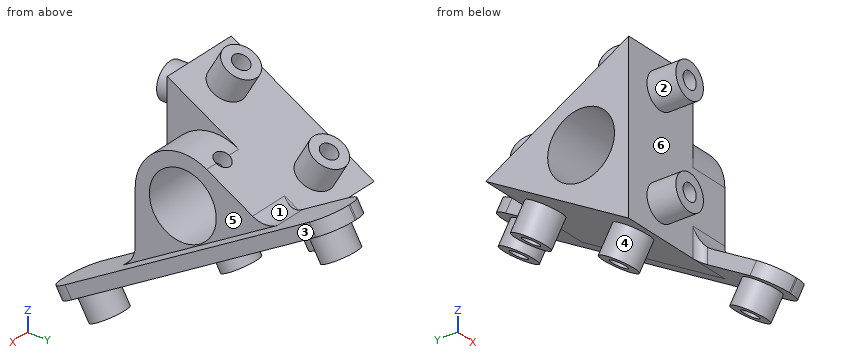
```python
from build123d import *

# Parameters (mm, degrees)
SKETCH_R           = 4.05
PAD_DEPTH          = 15
SKETCH001_R        = 2.15
SKETCH001_R_2      = 1.025
PAD001_DEPTH       = 3.5
POLARPATTERN_COUNT = 3
POLARPATTERN_ANGLE = 240
SKETCH002_R        = 1
POCKET_DEPTH       = 5
SKETCH003_W        = 40
SKETCH003_H        = 6
PAD002_DEPTH       = 1.6
SKETCH004_R        = 2.15
SKETCH004_R_2      = 1.025
PAD003_DEPTH       = 3
POCKET001_DEPTH    = 5
FILLET_R           = 3
FILLET001_R        = 2.9
FILLET002_R        = 1
FILLET003_R        = 1


with BuildPart() as part:
    # Sketch → Pad (new body)
    with BuildSketch(Plane.YZ):
        Polygon((-5.7735026919, 10), (-5.7735026919, -10), (11.5470053838, 0), align=None)
        Circle(SKETCH_R, mode=Mode.SUBTRACT)
    extrude(amount=PAD_DEPTH)

    # Sketch001 (on Face1 of Pad) → Pad001 (join)
    with BuildSketch(Plane(origin=(0, -5.7735026919, 0), x_dir=(0, 0, -1), z_dir=(0, -1, 0))):
        with Locations((6.15, 5)):
            Circle(SKETCH001_R)
        with Locations((6.15, 5)):
            Circle(SKETCH001_R_2, mode=Mode.SUBTRACT)
        with Locations((-6.15, 5)):
            Circle(SKETCH001_R)
        with Locations((-6.15, 5)):
            Circle(SKETCH001_R_2, mode=Mode.SUBTRACT)
    pad001 = extrude(amount=PAD001_DEPTH)

    # PolarPattern: Pad001 ×3 about axis
    polarpattern_axis = Axis((0, 0, 0), (1, 0, 0))
    for i in range(1, POLARPATTERN_COUNT):
        add(pad001.rotate(polarpattern_axis, i * POLARPATTERN_ANGLE / (POLARPATTERN_COUNT - 1)))

    # Sketch002 (on Face2 of PolarPattern) → Pocket (cut)
    with BuildSketch(Plane(origin=(0, 2.8867513459, 5), x_dir=(0, -0.8660254038, 0.5), z_dir=(0, 0.5, 0.8660254038))):
        with Locations((0, 12.5)):
            Circle(SKETCH002_R)
    extrude(amount=-POCKET_DEPTH, mode=Mode.SUBTRACT)

    # Sketch003 (on Face5 of Pocket) → Pad002 (join)
    with BuildSketch(Plane(origin=(0, 2.8867513459, -5), x_dir=(0, 0.8660254038, 0.5), z_dir=(0, 0.5, -0.8660254038))):
        with Locations((0, 14)):
            Rectangle(SKETCH003_W, SKETCH003_H)
    extrude(amount=-PAD002_DEPTH)

    # Sketch004 (on Face14 of Pad002) → Pad003 (join)
    with BuildSketch(Plane(origin=(0, 2.8867513459, -5), x_dir=(0, 0.8660254038, 0.5), z_dir=(0, 0.5, -0.8660254038))):
        with Locations((-16.2, 14)):
            Circle(SKETCH004_R)
        with Locations((-16.2, 14)):
            Circle(SKETCH004_R_2, mode=Mode.SUBTRACT)
        with Locations((16.2, 14)):
            Circle(SKETCH004_R)
        with Locations((16.2, 14)):
            Circle(SKETCH004_R_2, mode=Mode.SUBTRACT)
    extrude(amount=PAD003_DEPTH)

    # Sketch005 (on Face6 of Pad003) → Pocket001 (cut)
    with BuildSketch(Plane.YZ.offset(15)):
        with BuildLine():
            Line((-5.7735026919, 0), (-5.7735026919, 10))
            Line((-5.7735026919, 10), (2.8867345187, 5.0000097152))
            ThreePointArc((2.8867345187, 5.0000097152), (-2.8867597595, 4.9999951424), (-5.7735026919, 0))
        make_face()
    extrude(amount=-POCKET001_DEPTH, mode=Mode.SUBTRACT)

    # Fillet
    fillet_edges = [part.edges().sort_by_distance(p)[0] for p in [
        (13, 9.947005, 0.92376),
        (13, -5.773503, -8.152479),
    ]]
    fillet(fillet_edges, radius=FILLET_R)

    # Fillet001
    fillet001_edges = [part.edges().sort_by_distance(p)[0] for p in [
        (17, -14.833757, -14.30718),
        (11, -14.833757, -14.30718),
        (17, 19.807259, 5.69282),
        (11, 19.807259, 5.69282),
    ]]
    fillet(fillet001_edges, radius=FILLET001_R)

    # Fillet002
    fillet002_edges = [part.edges().sort_by_distance(p)[0] for p in [
        (11, -5.773503, -9.07624),
        (11, -5.773503, -7.286454),
    ]]
    fillet(fillet002_edges, radius=FILLET002_R)

    # Fillet003
    fillet003_edges = [part.edges().sort_by_distance(p)[0] for p in [
        (11, 9.197005, 1.356773),
        (11, 10.747005, 0.46188),
    ]]
    fillet(fillet003_edges, radius=FILLET003_R)


solid = part.part
```
Geometry check sheet. Reference: the model listing, model coordinates, mm. Face numbers are marked on the shaded views. A direction names the side the tool comes from. Give positions to 0.01 mm unless a question says otherwise; leave off trailing zeros. Loops run counter-clockwise (first coordinate to the right, second up) from the corner with the lowest first, then second, coordinate; pieces in that order, holes last. Notation, with made-up numbers: M 18.5,7.5 L 51.5,7.5 A17 cw 51.5,16.5 Z; hole C 65.5,-24.5 d6. An arc over 180 degrees is marked long. Write item = value, one per line. Start each with the question number.
1. Section check C-C, the plane x = 2. Enter the section's corners in (y, z).
2. Go/stop test with flat-tipped pins: P1, Ø1, axis at y = 3.5, z = -7.5, coming from the -X side; P2, Ø3.5, axis at x = 5, z = -5.5, coming from the -Y side; P3, Ø1.2, axis at x = 5, z = -6.15, coming from the -Y side; P4, Ø1.5, axis at x = 4, z = -12.5, coming from the +Y side. Record where each tip stops, or that it passes through.
3. Thickness scan on probe 1 along X at (y, z) = (-8.5, -6.15) (3 decimals); probe 2 along X at (y, z) = (-7, 4.5); probe 3 along X at (y, z) = (-0.5, 4.5). Record the ranges inside material, lowest first.
4. Draft check along Y on the marked faces 4, 5 and 6. Enter one of: +Y half, -Y half, draft (parallel to the pull), parting line (faces both ways), or undercut.
5. Section check A-A, the plane x = 6.5. Enter the section's corners in (y, z), plus the area to 3 significant figures.
6. Section check B-B, the plane y = 13. Enter the section's corners in (x, z), plus the area to 3 significant figures.
7. Tool access check on the marked faces 1, 2 and 3. Record the directions out of +Z, -Z, +X, -X, +Y, -Y that give a thin tool (end or side, any length) a straight path to the whole face; none if there is none.
Values follow:
q1.outline = M -5.77,-10 L 11.55,0 L -5.77,10 Z; hole C 0,0 d8.1
q2.P1 = through
q2.P2 = -9.27
q2.P3 = -5.77
q2.P4 = -1.8
q3.probe_1 = 2.85 to 3.975, 6.025 to 7.15
q3.probe_2 = 3.62 to 6.38
q3.probe_3 = 0 to 15
q4.face_4 = undercut
q4.face_5 = draft
q4.face_6 = -Y half
q5.outline = M -9.27,-7.69 L -5.77,-7.69 L -5.77,-10 L -3.77,-8.85 L -2.02,-11.88 L 0.64,-10.34 L -1.11,-7.3 L 6.88,-2.7 L 8.63,-5.73 L 11.3,-4.19 L 9.55,-1.15 L 11.55,0 L 9.55,1.15 L 11.3,4.19 L 8.63,5.73 L 6.88,2.7 L -1.11,7.3 L 0.64,10.34 L -2.02,11.88 L -3.77,8.85 L -5.77,10 L -5.77,7.69 L -9.27,7.69 L -9.27,4.61 L -5.77,4.61 L -5.77,-4.61 L -9.27,-4.61 Z; hole C 0,0 d8.1
q5.area = 186 mm^2
q6.outline = M 11,0.84 L 17,0.84 L 17,2.69 L 11,2.69 Z
q6.area = 11.1 mm^2
q7.face_1 = +Z, +X
q7.face_2 = -Y
q7.face_3 = +Z, -Z, +X, +Y, -Y
